Study the drawing (mm; zero at the part's minimum x, y, z) and answer. A direction names the side the tool comes from. Coordinates: 2 decimals unless noted, no trailing zeros. Loops run counter-clockwise (first coordinate to the right, second up) from the corner with the lowest first, then second, coordinate; pieces in that order, holes last. Notation, with made-up numbers: (67, -38.5) -> (79, -38.5) arc R19 cw to (79, -26.5) -> close; hole circle Ø2 at (-21, 7.5). An arc over 180 degrees is marked (long way). Answer as a JSON object with one key per item and string values. Group by question number.
Q1. Each of these flat-tipped pins is pushed along its axis until it touches: P1, Ø12, axis at y = 10, z = 57, coming from the +X side; P2, Ø12, axis at x = 23.5, y = 24.5, coming from the +Z side; P3, Ø12, axis at y = 8.5, z = 11.5, coming from the +X side. Where does it stop, or does it pass through?
Q2. The part is cut by section A-A on x = 32. Write down the section's boundary in (y, z), and give its area (3 significant figures).
Q3. For the marked faces 1, 2 and 3, determine the directions among +Z, -Z, +X, -X, +Y, -Y from which every point of the face is accessible in a straight line to the end or side of a thin tool.
Q4. The part is cut by section D-D on y = 6.5. Write down the section's boundary in (x, z), and give its area (3 significant figures).
Q5. The part is cut by section B-B on z = 5. Write down the section's boundary in (x, y), and give its area (3 significant figures).
Q6. The part is cut by section C-C on z = 34. Write down the section's boundary in (x, y).
Q7. Straight lines are drawn through the part: line 1 along Z through (x, y) = (32, 1.05); line 2 along Y through (x, z) = (25, 95); line 3 along X through (y, z) = (18, 68.5). For each, find the intervals that lie inside material, in ascending order. Write a range as [from, to].
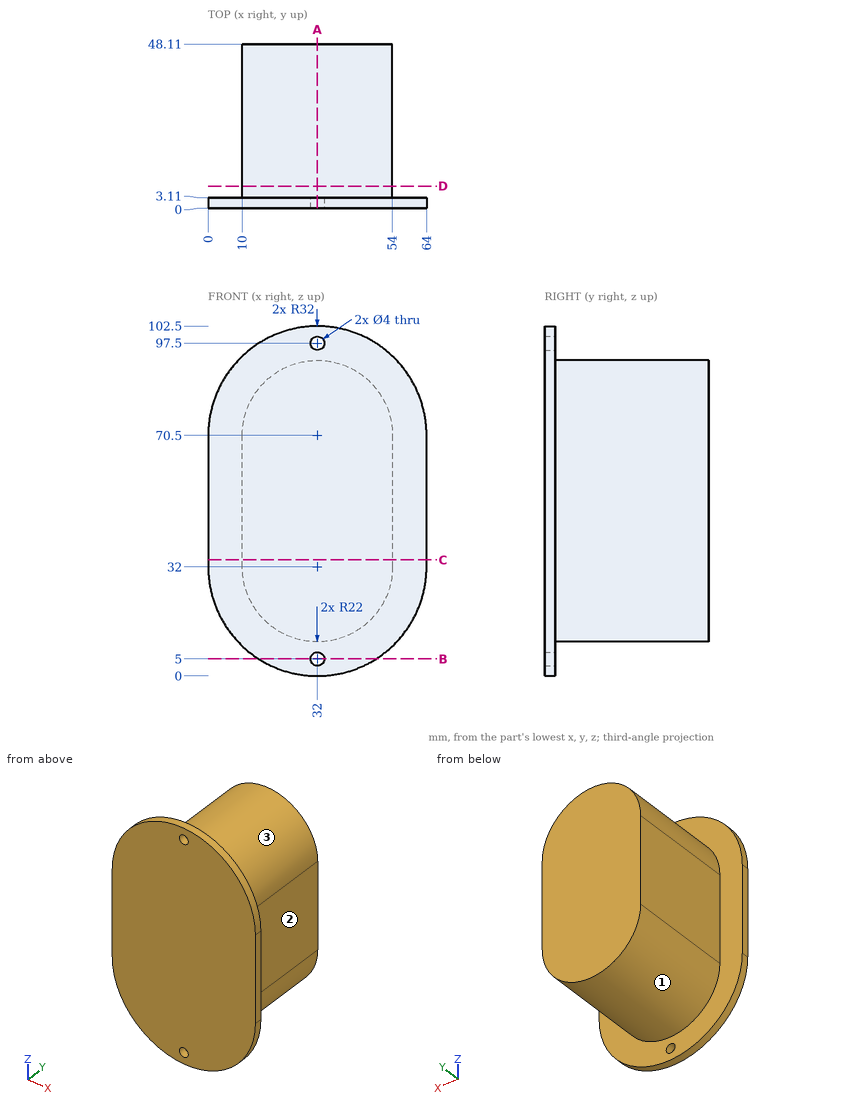
Final values:
{
 "1": {"P1": "stops at x = 54", "P2": "stops at z = 92.36", "P3": "stops at x = 58.55"},
 "2": {"outline": "(0, 0) -> (3.11, 0) -> (3.11, 3) -> (0, 3) -> close; (0, 7) -> (3.11, 7) -> (3.11, 10) -> (48.11, 10) -> (48.11, 92.5) -> (3.11, 92.5) -> (3.11, 95.5) -> (0, 95.5) -> close; (0, 99.5) -> (3.11, 99.5) -> (3.11, 102.5) -> (0, 102.5) -> close", "area": "4,010 mm2"},
 "3": {"face 1": "-Z, +Y", "face 2": "+Z, -Z, +X, +Y", "face 3": "+Z, +Y"},
 "4": {"outline": "(10, 32) arc R22 ccw to (54, 32) -> (54, 70.5) arc R22 ccw to (10, 70.5) -> close", "area": "3,210 mm2"},
 "5": {"outline": "(14.82, 0) -> (30, 0) -> (30, 3.11) -> (14.82, 3.11) -> close; (34, 0) -> (49.18, 0) -> (49.18, 3.11) -> (34, 3.11) -> close", "area": "94.4 mm2"},
 "6": {"outline": "(0, 0) -> (64, 0) -> (64, 3.11) -> (54, 3.11) -> (54, 48.11) -> (10, 48.11) -> (10, 3.11) -> (0, 3.11) -> close"},
 "7": {"line 1": "z = [0, 3], [7, 95.5], [99.5, 102.5]", "line 2": "y = [0, 3.11]", "line 3": "x = [10, 54]"}
}
